Build history of the part. All positions in model axes, mm. A direction names the side the tool comes from. Give positions to 0.01 mm unless a question says otherwise; leave off trailing zeros. Order: outer loops, then holes, each group sorted by start corner. A loop starts at its lowest first (then second) coordinate and runs counter-clockwise, first axis right, second up. Notation, with made-up numbers: M 23.25,-4 L 77.25,-4 A21 cw 77.25,15 Z; hole C -26,89 d1. An arc over 180 degrees is marked long. One line per item, written item: value. Start each with the question number.
from build123d import *

# Parameters (mm, degrees)
SKETCH1_W                   = 515.597416032
SKETCH1_H                   = 317.102213092
BOSS_EXTRUDE1_DEPTH         = 6
CUT_EXTRUDE_THIN1_START     = -6
CUT_EXTRUDE_THIN1_OUTLINE_W = 515.597416032
CUT_EXTRUDE_THIN1_OUTLINE_H = 317.102213092
CUT_EXTRUDE_THIN1_DEPTH     = 6


# Read off the part's stored shape, not the designer's step: Cut-Extrude-Thin1
with BuildPart() as part:
    # Sketch1 → Boss-Extrude1 (new body)
    with BuildSketch(Plane(origin=(0, 0, 0), x_dir=(1, 0, 0), z_dir=(0, 1, 0))):
        Rectangle(SKETCH1_W, SKETCH1_H)
    extrude(amount=BOSS_EXTRUDE1_DEPTH)

    # Cut-Extrude-Thin1 outline → Cut-Extrude-Thin1 (cut)
    with BuildSketch(Plane(origin=(0, 6, 0), x_dir=(1, 0, 0), z_dir=(0, 1, 0)).offset(CUT_EXTRUDE_THIN1_START)):
        Rectangle(CUT_EXTRUDE_THIN1_OUTLINE_W, CUT_EXTRUDE_THIN1_OUTLINE_H)
        with BuildLine():
            add(Edge.make_bspline(
                [(84.819466733, 25.244885548), (84.821389699, 29.41155314), (84.819617483, 33.578221619), (84.819636894, 37.744889655), (84.819695129, 50.244893831), (84.819695129, 62.744898008), (84.819695129, 75.244902185)],
                knots=[0, 0, 0, 0, 0.012500004, 0.012500004, 0.012500004, 0.050000017, 0.050000017, 0.050000017, 0.050000017], degree=3))
            Line((84.819466733, 25.244885548), (67.579926926, 25.244885548))
            Line((67.579926926, 25.244885548), (67.579926926, 31.244916231))
            Line((67.579926926, 31.244916231), (27.06992581, 31.244916231))
            Line((27.06992581, 31.244916231), (27.06992581, 25.244885548))
            Line((27.06992581, 25.244885548), (-13.420075307, 25.244885548))
            Line((-13.420075307, 25.244885548), (-13.420075307, 31.244916231))
            Line((-13.420075307, 31.244916231), (-41.87677177, 31.244916231))
            Line((-41.87677177, 31.244916231), (-41.87677177, 54.984916885))
            Line((-41.87677177, 54.984916885), (-41.875093181, 54.984916885))
            Line((-41.875093181, 54.984916885), (-41.875093181, 95.494918002))
            Line((-41.875093181, 95.494918002), (-41.87677177, 95.494918002))
            Line((-41.87677177, 95.494918002), (-41.87677177, 119.234918656))
            Line((-41.87677177, 119.234918656), (-13.420075307, 119.234918656))
            Line((-13.420075307, 119.234918656), (-13.420075307, 125.234918822))
            Line((-13.420075307, 125.234918822), (27.06992581, 125.234918822))
            Line((27.06992581, 125.234918822), (27.06992581, 119.234918656))
            Line((27.06992581, 119.234918656), (67.579926926, 119.234918656))
            Line((67.579926926, 119.234918656), (67.579926926, 125.234918822))
            Line((67.579926926, 125.234918822), (108.069928043, 125.234918822))
            Line((108.069928043, 125.234918822), (108.069928043, 119.234918656))
            Line((108.069928043, 119.234918656), (148.579929159, 119.234918656))
            Line((148.579929159, 119.234918656), (148.579929159, 125.234918822))
            Line((148.579929159, 125.234918822), (189.069930275, 125.234918822))
            Line((189.069930275, 125.234918822), (189.069930275, 119.234918656))
            Line((189.069930275, 119.234918656), (217.526162193, 119.234918656))
            Line((217.526162193, 119.234918656), (217.526162193, 95.494918002))
            Line((217.526162193, 95.494918002), (217.524917632, 95.494918002))
            Line((217.524917632, 95.494918002), (217.524917632, 54.984916885))
            Line((217.524917632, 54.984916885), (217.526162193, 54.984916885))
            Line((217.526162193, 54.984916885), (217.526162193, 31.244916231))
            Line((217.526162193, 31.244916231), (189.069930275, 31.244916231))
            Line((189.069930275, 31.244916231), (189.069930275, 25.244885548))
            Line((189.069930275, 25.244885548), (148.579929159, 25.244885548))
            Line((148.579929159, 25.244885548), (148.579929159, 31.244916231))
            Line((148.579929159, 31.244916231), (108.069928043, 31.244916231))
            Line((108.069928043, 31.244916231), (108.069928043, 25.244885548))
            Line((108.069928043, 25.244885548), (90.829695294, 25.244885548))
            Line((90.829695294, 25.244885548), (90.829695294, 75.244902185))
            Line((90.829695294, 75.244902185), (84.819695129, 75.244902185))
        make_face(mode=Mode.SUBTRACT)
    extrude(amount=CUT_EXTRUDE_THIN1_DEPTH, mode=Mode.SUBTRACT)


solid = part.part
1) Slice it at A-A (x = 195). List the corners of the cut face in (y, z).
2) Drill centre lines: line 1 (X direction, y = 3.5, z = -31); line 2 (X direction, y = 3.25, z = -62); line 3 (Z direction, x = -17, y = 2.25). Where is each one in solid material? Low to high.
3) Tool access for faces 4 (the flat face through (-13.42, 3, -28)), 5 (the flat face through (189.07, 3, -28)), 6 (the flat face through (48, 3, -31.245)): list every direction of +Z, -Z, +X, -X, +Y, -Y with a clear straight run to the whole face (end or side of a thin tool).
4) Drop flat-ended pins along their axis: P1, Ø1.8, axis at x = 57, y = 3.5, coming from the +Z side; P2, Ø1.8, axis at y = 3, z = -29.5, coming from the +X side. Give the stop position or say it passes through.
5) Pull direction X, two halves, no side cores. Call faces 1 (the flat face through (100, 3, -25.245)), 2 (the flat face through (217.526, 3, -108)), 3 (the flat face through (27.07, 3, -122)): pulls with the +X half, pulls with the -X half, needs draft (parallel to the pull), parting line crosses it, or undercut.
Results list:
1. outline: M 0,-119.23 L 6,-119.23 L 6,-31.24 L 0,-31.24 Z
2. line 1: x = -13.42 to 27.07, 67.58 to 84.82, 90.83 to 108.07, 148.58 to 189.07
2. line 2: x = -41.88 to 84.82, 90.83 to 217.52
2. line 3: z = -119.23 to -31.24
3. face 4: +Z, -X, +Y, -Y
3. face 5: +Z, +X, +Y, -Y
3. face 6: +Z, +Y, -Y
4. P1: stops at z = -31.24
4. P2: stops at x = 189.07
5. face 1: needs draft
5. face 2: pulls with the +X half
5. face 3: undercut
